from build123d import *

# Parameters (mm, degrees)
SURFACE_EXTRUDE1_1_BACK  = 10
SURFACE_EXTRUDE1_1_DEPTH = 10
THICKEN1_T1              = 3


with BuildPart() as body_1:
    # Surface-Extrude1: a surface, the sketch's curves swept straight by 10 mm
    with BuildLine(Plane.XY.offset(-SURFACE_EXTRUDE1_1_BACK), mode=Mode.PRIVATE) as surface_extrude1_1_path:
        Line((-22.283440581, 8.913376232), (34.716559419, 151.413376232))
        ThreePointArc((34.716559419, 151.413376232), (65.913376232, 164.783440581), (79.283440581, 133.586623767))
        Line((79.283440581, 133.586623767), (22.283440581, -8.913376232))
        ThreePointArc((22.283440581, -8.913376232), (-8.913376232, -22.283440581), (-22.283440581, 8.913376232))
    surface_extrude1_1 = Shell.extrude(surface_extrude1_1_path.wire(), (0 * SURFACE_EXTRUDE1_1_DEPTH, 0 * SURFACE_EXTRUDE1_1_DEPTH, 1 * SURFACE_EXTRUDE1_1_DEPTH))
    add(Solid.thicken(surface_extrude1_1, THICKEN1_T1))


solid = body_1.part
Geometry check sheet. Reference: the model listing, model coordinates, mm. A direction names the side the tool comes from. Round coordinates to 2 decimals unless told otherwise and drop trailing zeros. Order: outer loops, then holes, each group sorted by start corner. A loop starts at its lowest first (then second) coordinate and runs counter-clockwise, first axis right, second up. Notation, with made-up numbers: M 32,6 L 74,6 A19 ccw 74,10 Z; hole C 60.25,-4 d1. An arc over 180 degrees is marked long. Answer in a Markdown table with one row per item.
(1) Sectioned sample at B-B, the plane y = 135.5. Record the cut outline in (x, z), and give its area (3 significant figures).
Responses:
| item | result |
|---|---|
| outline | M 25.12,-10 L 28.35,-10 L 28.35,0 L 25.12,0 Z; M 79.96,-10 L 83.08,-10 L 83.08,0 L 79.96,0 Z |
| area | 63.5 mm² |
(2) Scan lines: probe 1 along X at (y, z) = (7, -3.5); probe 2 along X at (y, z) = (-1.5, -3.5); probe 3 along Y at (x, z) = (48, -7.25). Record each from-to range of solid material in increasing order. Write a range as from..to.
Responses:
| item | result |
|---|---|
| probe 1 | x = -26.08..-22.96, 28.65..31.88 |
| probe 2 | x = -26.96..-23.95, 25.25..28.48 |
| probe 3 | y = 47.3..55.38, 164.75..167.96 |
(3) Sectioned sample at C-C, the plane x = -9.5. Record the cut outline in (y, z), and give its area (3 significant figures).
Responses:
| item | result |
|---|---|
| outline | M -25.27,-10 L -22.04,-10 L -22.04,0 L -25.27,0 Z; M 40.87,-10 L 48.95,-10 L 48.95,0 L 40.87,0 Z |
| area | 113 mm² |
(4) Tool access check on faces 1 (the face through (8, 86, -10)), 2 (the face through (51.18, 63.33, -5.07)). Record the directions out of +Z, -Z, +X, -X, +Y, -Y that give a thin tool (end or side, any length) a straight path to the whole face; none if there is none.
Responses:
| item | result |
|---|---|
| face 1 | -Z, +X, -X, +Y, -Y |
| face 2 | +Z, -Z |
(5) Draft check along Y on faces 3 (the face through (5.82, 79.17, -5.07)), 4 (the face through (66.474, 167.783, -5.07)), 5 (the face through (3.03, 80.28, -5.07)). Enter one of: released by +Y, released by -Y, zero draft, split by the parting line, or undercut.
Responses:
| item | result |
|---|---|
| face 3 | undercut |
| face 4 | split by the parting line |
| face 5 | released by +Y |
(6) Go/stop test with flat-tipped pins: P1, Ø1, axis at y = 40.5, z = -2, coming from the +X side; P2, Ø5, axis at y = 28.5, z = -7.5, coming from the -X side; P3, Ø6, axis at x = 65.5, z = -7, coming from the -Y side. Record where each tip stops, or that it passes through.
Responses:
| item | result |
|---|---|
| P1 | stops at x = 45.48 |
| P2 | stops at x = -18.68 |
| P3 | stops at y = 83.55 |
